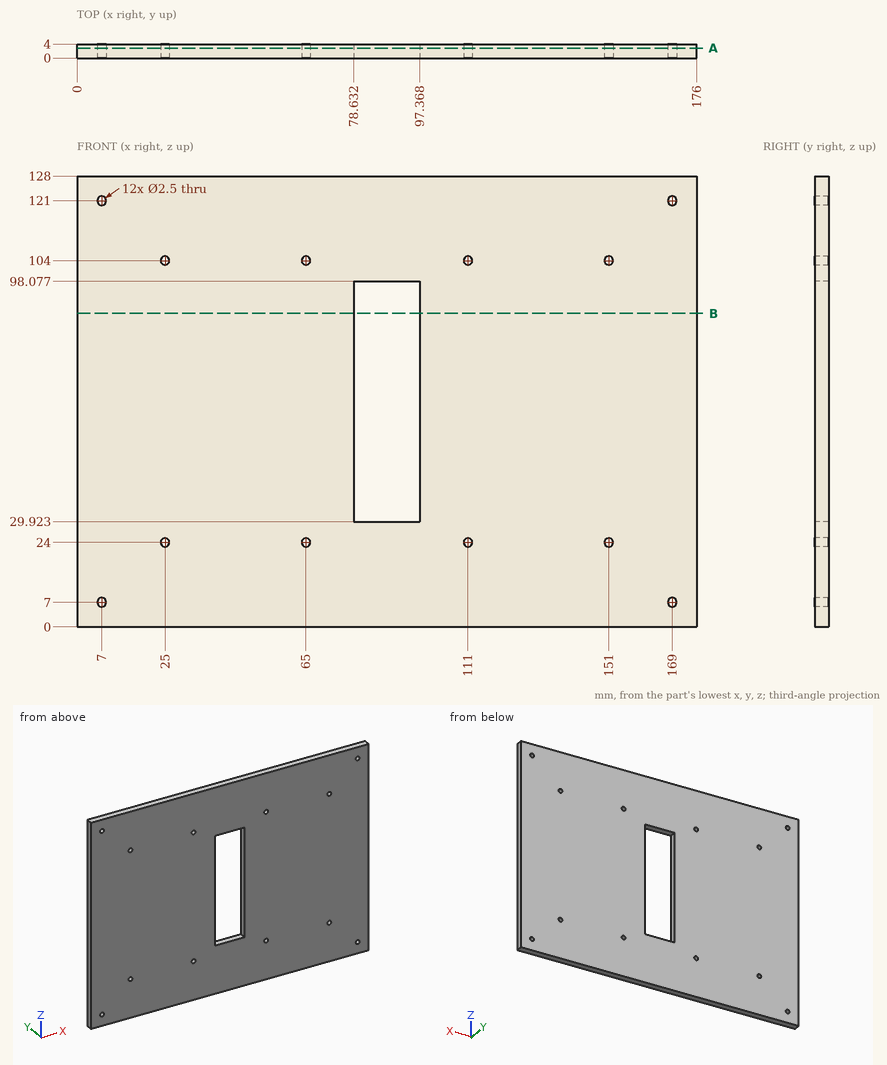
For this review, use the dimensioned drawing (mm, ordinates from the lowest corner) and the shaded views. Coordinates: 2 decimals unless noted, no trailing zeros. Write each loop counter-clockwise with the first axis right and the second up, starting at its lowest first coordinate (ties: lowest second). Pieces come first, ordered by that corner, then holes. Notation, with made-up numbers: (8, -2.75) - (63, -2.75) arc R24 ccw to (63, 20.25) - close; hole circle Ø9 at (39, -13). An arc over 180 degrees is marked (long way). Answer in a Markdown table with one row per item. Add a question column.
Q1. Consider section B-B on z = 89. Give the boundary of the cut face in (x, y).
Q2. Consider section A-A on y = 2.8. Give the number of separate pieces and of enclosed holes in the cut face, then the cut area to 3 significant figures.
Q3. To check wall thickness, follow line 1 along X through (y, z) = (1.55, 24); line 2 along X through (y, z) = (2.15, 121); line 3 along Z through (x, y) = (111, 2.45). State the ranges of each line that lie inside material, in increasing order. Write a range as from..to.
Q4. Clearance check with flat-ended pins moving along their axes: pin 1 (1 mm diameter, centred on x = 92.5, z = 24, fed in from -Y); pin 2 (2 mm diameter, centred on x = 7, z = 121, fed in from -Y). State where each tip first meets the part, or that it passes through.
Answers below:
| question | item | result |
|---|---|---|
| 1 | outline | (0, 0) - (78.63, 0) - (78.63, 4) - (0, 4) - close; (97.37, 0) - (176, 0) - (176, 4) - (97.37, 4) - close |
| 2 | separate pieces | 1 |
| 2 | enclosed holes | 13 |
| 2 | area | 21,200 mm² |
| 3 | line 1 | 0..23.75, 26.25..63.75, 66.25..109.75, 112.25..149.75, 152.25..176 |
| 3 | line 2 | 0..5.75, 8.25..167.75, 170.25..176 |
| 3 | line 3 | 0..22.75, 25.25..102.75, 105.25..128 |
| 4 | pin 1 | y = 0 |
| 4 | pin 2 | through |
